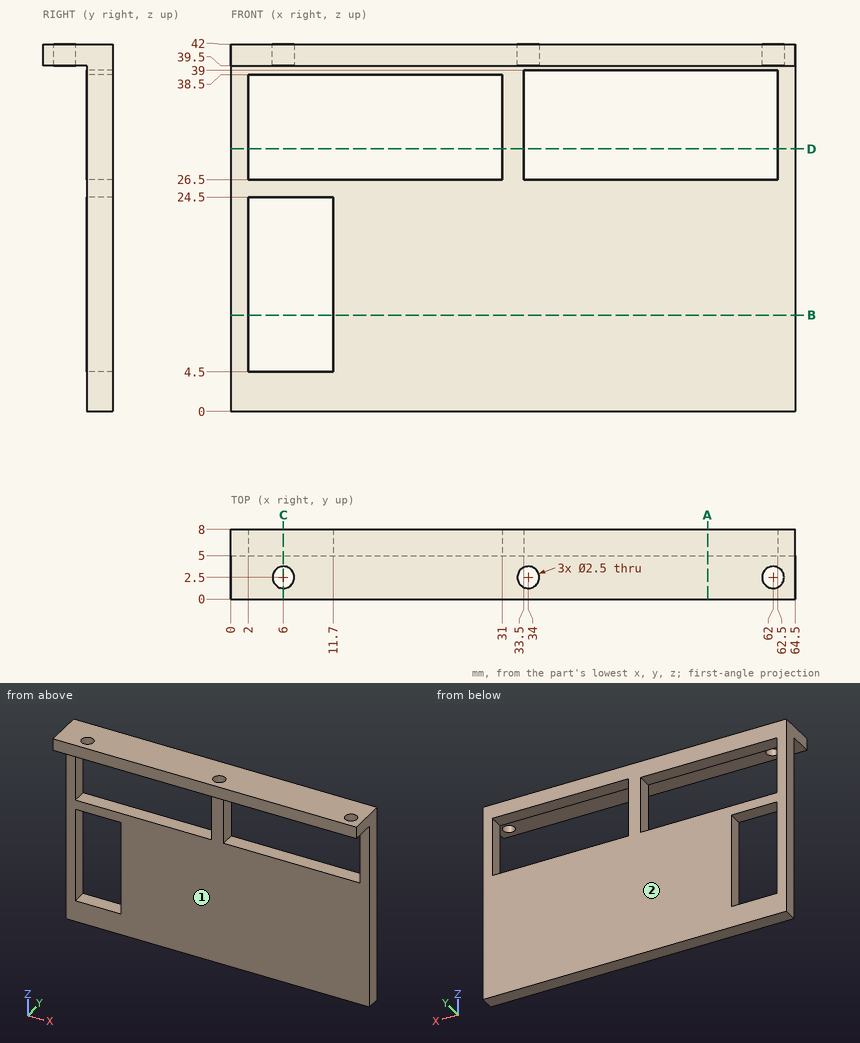
Can you work these out from the drawing? Everything is in mm from the part's minimum corner. A direction names the side the tool comes from. Round coordinates to 2 decimals unless told otherwise and drop trailing zeros. Order: outer loops, then holes, each group sorted by start corner. A loop starts at its lowest first (then second) coordinate and runs counter-clockwise, first axis right, second up. Notation, with made-up numbers: (30.25, -40) -> (57.25, -40) arc R26 ccw to (57.25, -21) -> close; hole circle Ø9 at (80.5, 31). An arc over 180 degrees is marked (long way). Return JSON: item names as keys, results as strings. Group by question number.
1. If we section it at D-D, the plane z = 30: Write out the boundary of the cut face in (x, y), then the cut area to 3 significant figures.
2. If we section it at B-B, the plane z = 11: Write out the boundary of the cut face in (x, y), then the cut area to 3 significant figures.
3. Which directions (+Z, -Z, +X, -X, +Y, -Y) give clear straight access to the entire face, cutting with the end or side of a thin tool? Please do the marked faces 1 and 2.
4. Will these pins go through, and if not, where does the flat tip stop? pin 1 (1.5 mm diameter, centred on x = 34, y = 2.5, fed in from -Z); pin 2 (4 mm diameter, centred on x = 50, z = 14, fed in from -Y).
5. If we section it at A-A, the plane x = 54.5: Write out the boundary of the cut face in (y, z).
6. If we section it at C-C, the plane x = 6: Write out the boundary of the cut face in (y, z).
7. I need wall thicknesses on line 1 (Z direction, x = 34, y = 7.5); line 2 (Y direction, x = 6, z = 40.8); line 3 (Z direction, x = 29.5, y = 6.75). Which ranges of each line are inside material? Lowest first, please. Write a range as [from, to].
Output values:
{
 "1": {"outline": "(0, 5) -> (2, 5) -> (2, 8) -> (0, 8) -> close; (31, 5) -> (33.5, 5) -> (33.5, 8) -> (31, 8) -> close; (62.5, 5) -> (64.5, 5) -> (64.5, 8) -> (62.5, 8) -> close", "area": "19.5 mm²"},
 "2": {"outline": "(0, 5) -> (2, 5) -> (2, 8) -> (0, 8) -> close; (11.7, 5) -> (64.5, 5) -> (64.5, 8) -> (11.7, 8) -> close", "area": "164 mm²"},
 "3": {"face 1": "-Z, +X, -X, -Y", "face 2": "+Z, -Z, +X, -X, +Y"},
 "4": {"pin 1": "through", "pin 2": "y = 5"},
 "5": {"outline": "(0, 39.5) -> (5, 39.5) -> (5, 39) -> (8, 39) -> (8, 42) -> (0, 42) -> close; (5, 0) -> (8, 0) -> (8, 26.5) -> (5, 26.5) -> close"},
 "6": {"outline": "(0, 39.5) -> (1.25, 39.5) -> (1.25, 42) -> (0, 42) -> close; (3.75, 39.5) -> (5, 39.5) -> (5, 38.5) -> (8, 38.5) -> (8, 42) -> (3.75, 42) -> close; (5, 0) -> (8, 0) -> (8, 4.5) -> (5, 4.5) -> close; (5, 24.5) -> (8, 24.5) -> (8, 26.5) -> (5, 26.5) -> close"},
 "7": {"line 1": "[0, 26.5], [39, 42]", "line 2": "[0, 1.25], [3.75, 8]", "line 3": "[0, 26.5], [38.5, 42]"}
}
